Drawing for the job (mm, zero at the part's lowest x, y, z). A direction names the side the tool comes from. Give positions to 0.01 mm unless a question says otherwise; leave off trailing zeros. Order: outer loops, then holes, each group sorted by start corner. A loop starts at its lowest first (then second) coordinate and runs counter-clockwise, first axis right, second up. Notation, with made-up numbers: (-23, 28) - (13, 28) arc R20 cw to (13, 35) - close; hole circle Ø10 at (79.25, 10). An arc over 180 degrees is marked (long way). One line per item, written item: value.
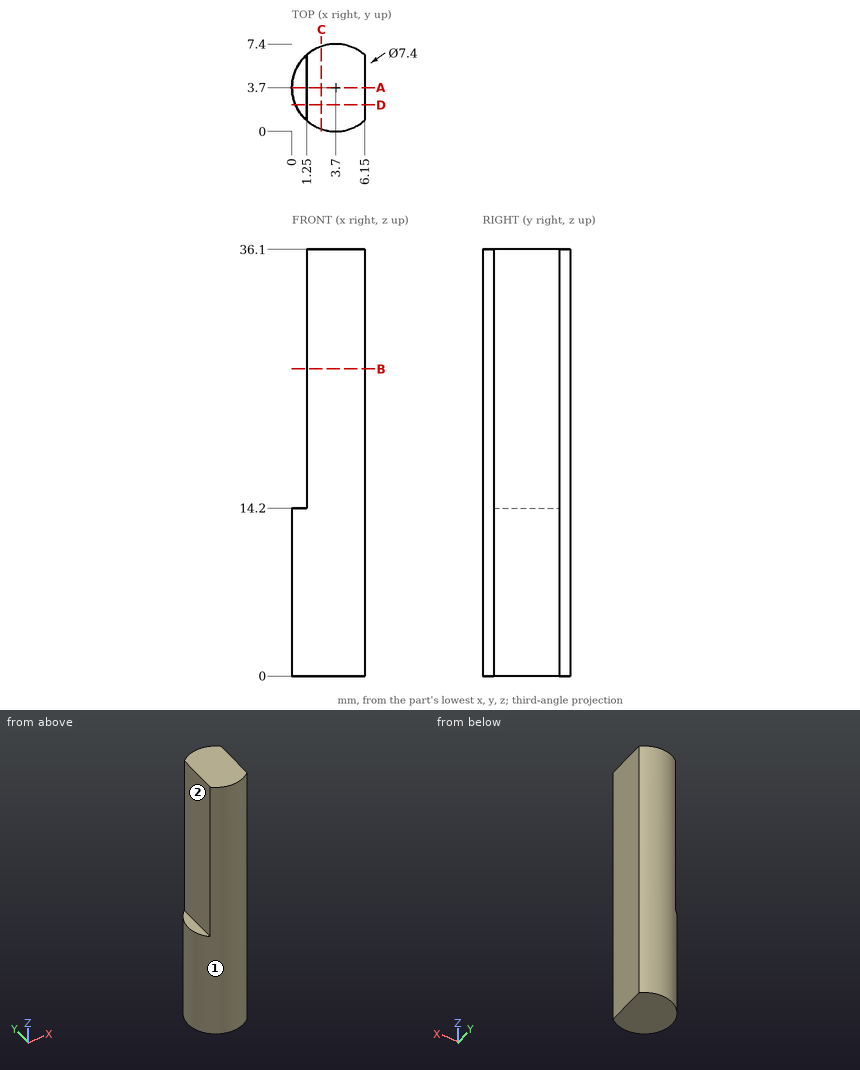
(1) Drill centre lines: line 1 (X direction, y = 4.25, z = 25); line 2 (Y direction, x = 1.25, z = 6); line 3 (Y direction, x = 5.25, z = 25.5). Where is each one in solid material? Low to high.
Completed:
line 1: 1.25 to 6.15
line 2: 0.93 to 6.47
line 3: 0.34 to 7.06
(2) Slice it at C-C, the plane x = 2.5. Give the cut face in (y, z), and give its area (3 significant figures).
Completed:
outline: (0.2, 0) - (7.2, 0) - (7.2, 36.1) - (0.2, 36.1) - close
area: 253 mm²
(3) Slice it at B-B, the plane z = 26. Give the cut face in (x, y).
Completed:
outline: (1.25, 0.93) arc R3.7 ccw to (6.15, 0.93) - (6.15, 6.47) arc R3.7 ccw to (1.25, 6.47) - close
(4) Slice it at A-A, the plane y = 3.7. Give the cut face in (x, z).
Completed:
outline: (0, 0) - (6.15, 0) - (6.15, 36.1) - (1.25, 36.1) - (1.25, 14.2) - (0, 14.2) - close
(5) Pin check, flat tips, straight feed: P1, Ø3, axis at y = 2.5, z = 24, coming from the -X side; P2, Ø1, axis at x = 5.5, z = 21.5, coming from the +Y side; P3, Ø3, axis at x = 2.5, z = 19.5, coming from the +Y side. Stop position of each tip, or through.
Completed:
P1: x = 1.25
P2: y = 7.16
P3: y = 7.4
(6) 3-axis set-ups, long thin cutter, end or side, ignore diameter. For the marked faces 1 and 2: which of +Z, -Z, +X, -X, +Y, -Y reach the whole face in a straight line?
Completed:
face 1: +Z, -Z
face 2: +Z, -X, +Y, -Y
(7) Slice it at D-D, the plane y = 2.25. Give the cut face in (x, z).
Completed:
outline: (0.3, 0) - (6.15, 0) - (6.15, 36.1) - (1.25, 36.1) - (1.25, 14.2) - (0.3, 14.2) - close
